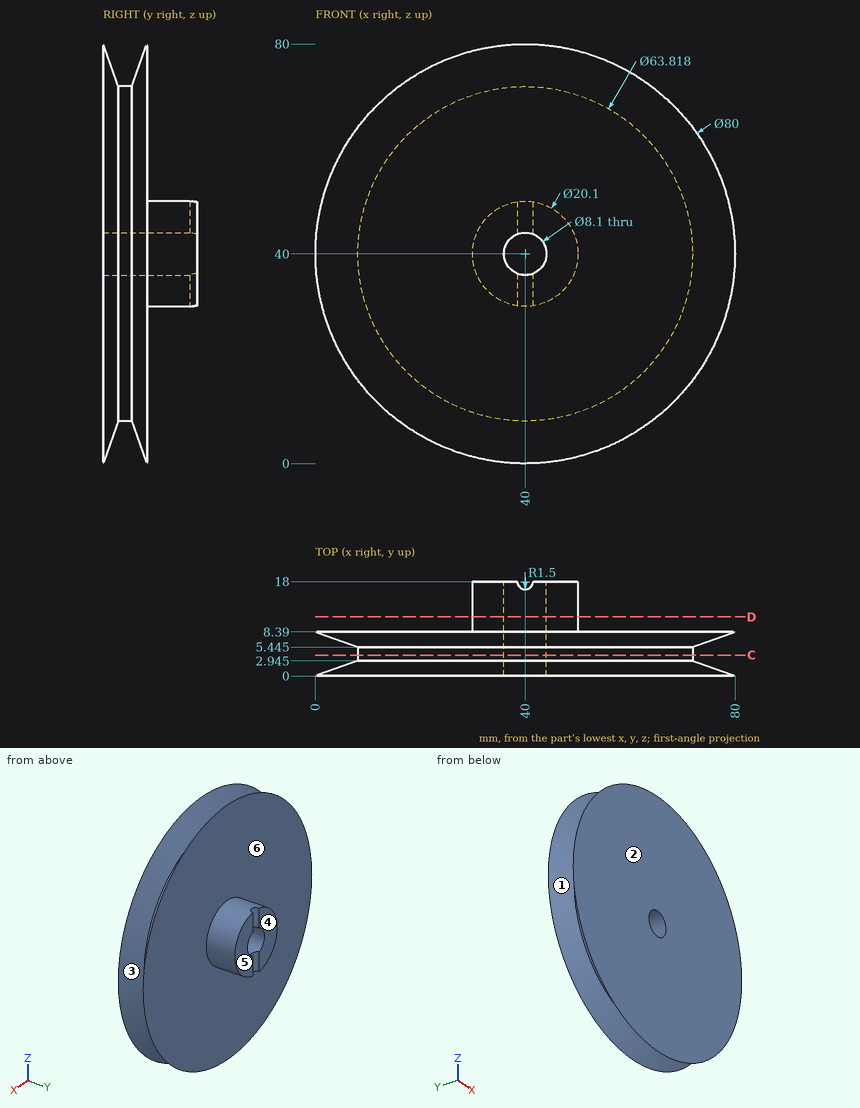
Geometry: see drawing. Coordinates: mm, zero at the bounding-box minimum. A direction names the side the tool comes from. Round coordinates to 2 decimals unless told otherwise and drop trailing zeros. Loops run counter-clockwise (first coordinate to the right, second up) from the corner with the lowest first, then second, coordinate; pieces in that order, holes last. Notation, with made-up numbers: (0, 55) - (35, 55) arc R31 cw to (35, 94) - close; hole circle Ø9 at (-12, 58.25). An arc over 180 degrees is marked (long way). Use CSV: the item, a comma, the result in double quotes.
Q1. Ray query, line 1 along Z through (x, y) = (40, 12); line 2 along Y through (x, z) = (44.5, 14). Return the intervals inside material, ascending.
Reported:
line 1,"29.95 to 35.95, 44.05 to 50.05"
line 2,"0 to 8.39"
Q2. Reachability of the marked faces 5 and 6 from +Z, -Z, +X, -X, +Y, -Y: full face, straight path, thin tool, end or side. Return the list, or none.
Reported:
face 5,"+Z, -Z, +X, -X, +Y"
face 6,"+Y"
Q3. Section query D-D, the plane y = 11.25. Output: boundary loops of the cut face in (x, z).
Reported:
outline,"circle Ø20.1 at (40, 40); hole circle Ø8.1 at (40, 40)"
Q4. Section query C-C, the plane y = 4. Output: boundary loops of the cut face in (x, z).
Reported:
outline,"circle Ø63.82 at (40, 40); hole circle Ø8.1 at (40, 40)"
Q5. Mould query, pull axis Y, two halves, no side actions, for the marked faces 1, 2, 3 and 4. Classes: pulls with the +Y half, pulls with the -Y half, needs draft (parallel to the pull), parting line crosses it, or undercut.
Reported:
face 1,"undercut"
face 2,"pulls with the -Y half"
face 3,"undercut"
face 4,"pulls with the +Y half"
Q6. Pin query (flat end, axial travel): pin 1 Ø2 at (y, z) = (14.5, 27) entering from +X; pin 2 Ø1 at (x, z) = (64, 12.5) entering from +Y. Return the tip coordinate at first contact, or that it passes through.
Reported:
pin 1,"through"
pin 2,"y = 8.39"
